For this review, take the finished solid that the model builds, in its own axes (mm). Coordinates: 2 decimals unless noted, no trailing zeros.
from build123d import *

# Parameters (mm, degrees)
SKETCH1_W           = 48.26
SKETCH1_H           = 63.5
BOSS_EXTRUDE1_DEPTH = 1.7
SKETCH3_R           = 3.175
SKETCH3_R_2         = 0.8382
SKETCH3_R_3         = 1.524
CUT_EXTRUDE1_DEPTH  = 80.775733152


with BuildPart() as part:
    # Sketch1 → Boss-Extrude1 (new body)
    with BuildSketch(Plane(origin=(0, 0, 0), x_dir=(1, 0, 0), z_dir=(0, 1, 0))):
        with Locations((24.13, 31.75)):
            Rectangle(SKETCH1_W, SKETCH1_H)
    extrude(amount=BOSS_EXTRUDE1_DEPTH)

    # Sketch3 → Cut-Extrude1 (cut, through all)
    with BuildSketch(Plane(origin=(0, 1.7, 0), x_dir=(1, 0, 0), z_dir=(0, 1, 0))):
        with Locations(Location((37.75456, 19.90598, 0), (0, 0, 270))):
            Circle(SKETCH3_R)
        with Locations(Location((36.9062, 11.4046, 0), (0, 0, 270))):
            Circle(SKETCH3_R)
        with Locations(Location((2.44856, 29.26842, 0), (0, 0, 270))):
            Circle(SKETCH3_R_2)
        with Locations(Location((4.98856, 29.26842, 0), (0, 0, 270))):
            Circle(SKETCH3_R_2)
        with Locations(Location((7.52856, 29.26842, 0), (0, 0, 270))):
            Circle(SKETCH3_R_2)
        with Locations(Location((10.06856, 29.26842, 0), (0, 0, 270))):
            Circle(SKETCH3_R_2)
        with Locations(Location((12.60856, 29.26842, 0), (0, 0, 270))):
            Circle(SKETCH3_R_2)
        with Locations(Location((15.14856, 29.26842, 0), (0, 0, 270))):
            Circle(SKETCH3_R_2)
        with Locations(Location((17.68856, 29.26842, 0), (0, 0, 270))):
            Circle(SKETCH3_R_2)
        with Locations(Location((20.22856, 29.26842, 0), (0, 0, 270))):
            Circle(SKETCH3_R_2)
        with Locations(Location((22.76856, 29.26842, 0), (0, 0, 270))):
            Circle(SKETCH3_R_2)
        with Locations(Location((25.30856, 29.26842, 0), (0, 0, 270))):
            Circle(SKETCH3_R_2)
        with Locations(Location((27.84856, 29.26842, 0), (0, 0, 270))):
            Circle(SKETCH3_R_2)
        with Locations(Location((30.38856, 29.26842, 0), (0, 0, 270))):
            Circle(SKETCH3_R_2)
        with Locations(Location((32.92856, 29.26842, 0), (0, 0, 270))):
            Circle(SKETCH3_R_2)
        with Locations(Location((35.46856, 29.26842, 0), (0, 0, 270))):
            Circle(SKETCH3_R_2)
        with Locations(Location((4.98856, 36.88842, 0), (0, 0, 270))):
            Circle(SKETCH3_R_2)
        with Locations(Location((7.52856, 36.88842, 0), (0, 0, 270))):
            Circle(SKETCH3_R_2)
        with Locations(Location((10.06856, 36.88842, 0), (0, 0, 270))):
            Circle(SKETCH3_R_2)
        with Locations(Location((12.60856, 36.88842, 0), (0, 0, 270))):
            Circle(SKETCH3_R_2)
        with Locations(Location((15.14856, 36.88842, 0), (0, 0, 270))):
            Circle(SKETCH3_R_2)
        with Locations(Location((17.68856, 36.88842, 0), (0, 0, 270))):
            Circle(SKETCH3_R_2)
        with Locations(Location((20.22856, 36.88842, 0), (0, 0, 270))):
            Circle(SKETCH3_R_2)
        with Locations(Location((22.76856, 36.88842, 0), (0, 0, 270))):
            Circle(SKETCH3_R_2)
        with Locations(Location((25.30856, 36.88842, 0), (0, 0, 270))):
            Circle(SKETCH3_R_2)
        with Locations(Location((27.84856, 36.88842, 0), (0, 0, 270))):
            Circle(SKETCH3_R_2)
        with Locations(Location((30.38856, 36.88842, 0), (0, 0, 270))):
            Circle(SKETCH3_R_2)
        with Locations(Location((32.92856, 36.88842, 0), (0, 0, 270))):
            Circle(SKETCH3_R_2)
        with Locations(Location((35.46856, 36.88842, 0), (0, 0, 270))):
            Circle(SKETCH3_R_2)
        with Locations(Location((2.44856, 36.88842, 0), (0, 0, 270))):
            Circle(SKETCH3_R_2)
        with Locations(Location((27.31008, 5.72008, 0), (0, 0, 270))):
            Circle(SKETCH3_R_3)
        with Locations(Location((5.0673, 58.34634, 0), (0, 0, 270))):
            Circle(SKETCH3_R_3)
        with Locations(Location((19.6723, 19.02714, 0), (0, 0, 270))):
            Circle(SKETCH3_R_2)
    extrude(amount=-CUT_EXTRUDE1_DEPTH, mode=Mode.SUBTRACT)


solid = part.part
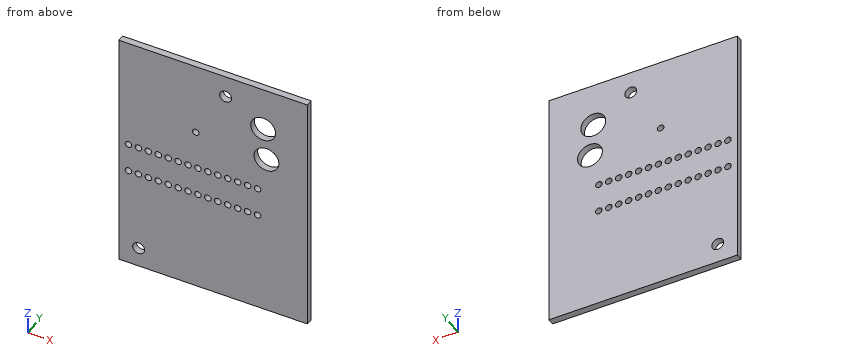
1. Take a section at A-A, the plane y = 0.9. Give the number of separate pieces and of enclosed holes in the cut face, plus the area to 3 significant figures.
Answer below:
separate pieces: 1
enclosed holes: 33
area: 2,920 mm2
2. To check wall thickness, follow L1, parallel to X at y = 0.2, z = -5.5; L2, parallel to Z at x = 10, y = 0.7; L3, parallel to Z at x = 25, y = 1. State the ranges of each line that lie inside material, in increasing order.
Answer below:
L1: x = 0 to 25.8, 28.82 to 48.26
L2: z = -63.5 to -37.72, -36.05 to -30.1, -28.43 to 0
L3: z = -63.5 to -37.67, -36.11 to -30.05, -28.49 to 0
3. Clearance check with a flat-ended pin moving along its axis: pin 1 Ø1 at (x, z) = (22.77, -29.27) entering from -Y. State where the tip first meets the part, or that it passes through.
Answer below:
pin 1: passes through
